The drawing under review shows one solid part. Ordinate dimensions are in mm from its lowest x, y, z. A direction names the side the tool comes from. Coordinates: 2 decimals unless noted, no trailing zeros. Write each loop counter-clockwise with the first axis right and the second up, starting at its lowest first coordinate (ties: lowest second). Pieces come first, ordered by that corner, then holes.
Q1. Insertion check: pin 1 (5 mm diameter, centred on x = 5.64, y = 5.64, fed in from -Z); pin 2 (2 mm diameter, centred on x = 2.5, z = 28.5, fed in from +Y); pin 3 (1.5 mm diameter, centred on y = 7.5, z = 12.5, fed in from -X). Each pin has a flat end and moves straight along its axis. Give the tip position at first contact, or say it passes through.
Q2. Take a section at B-B (y = 3.5). Give the boundary of the cut face in (x, z) (1 decimal), and give its area (3 significant figures).
Q3. Mouldability with a two-part tool opening along X and no side actions: class the marked faces 3, 4 and 5 as pulls with the +X half, pulls with the -X half, needs draft (parallel to the pull), parting line crosses it, or undercut.
Q4. Machinability: for the marked faces 1 and 2, which of the approach directions +Z, -Z, +X, -X, +Y, -Y give a long, thin tool a straight path to every point of the face, cutting with its end or side? Answer none if there is none.
Q5. Take a section at A-A (x = 7.25). Give the boundary of the cut face in (y, z) (1 decimal).
Q6. Take a section at D-D (z = 35). Give the boundary of the cut face in (x, y).
Q7. Take a section at C-C (z = 4.5). Give the boundary of the cut face in (x, y).
Q8. For probe 1 along Z at (x, y) = (0.75, 6.25); probe 2 along Z at (x, y) = (4.75, 7.5); probe 3 along Y at (x, z) = (6.75, 2), list the stretches that pass through material, from the lowest coordinate up.
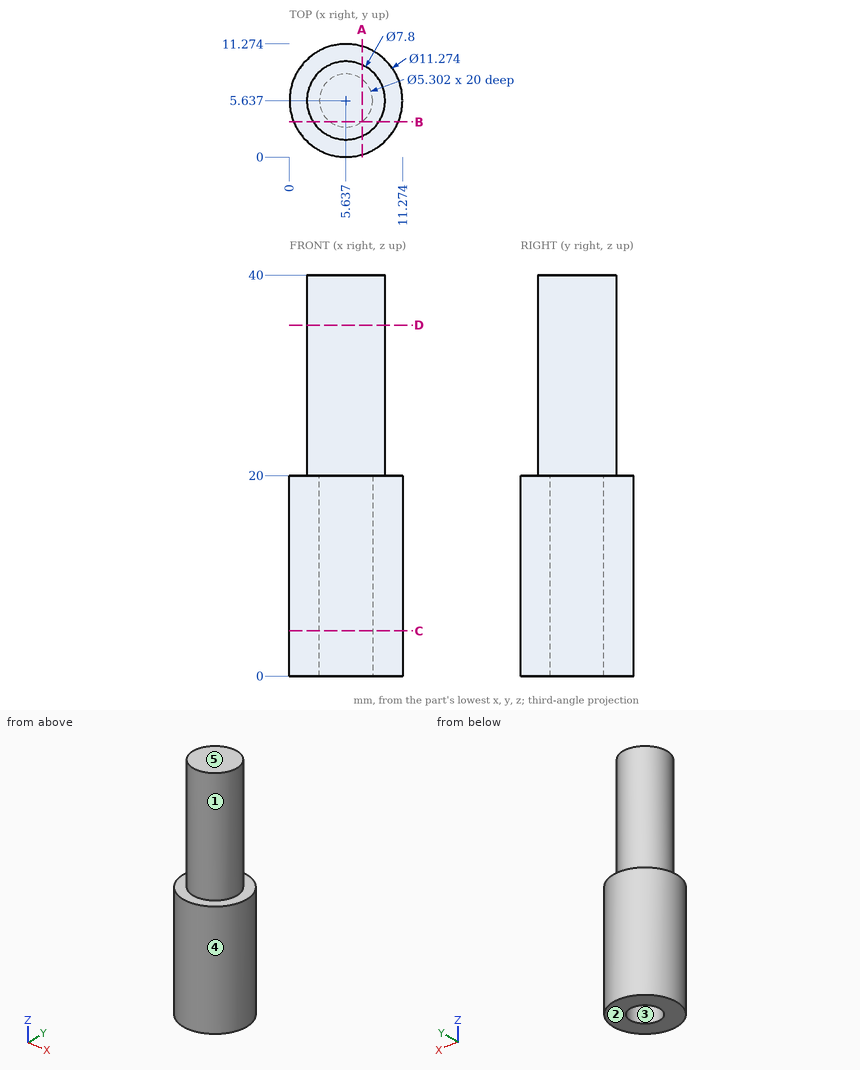
Response:
1. pin 1: stops at z = 20
1. pin 2: stops at y = 8.9
1. pin 3: stops at x = 0.11
2. outline: (0.4, 0) - (4.1, 0) - (4.1, 20) - (7.2, 20) - (7.2, 0) - (10.9, 0) - (10.9, 20) - (8.9, 20) - (8.9, 40) - (2.4, 40) - (2.4, 20) - (0.4, 20) - close
2. area: 276 mm2
3. face 3: undercut
3. face 4: parting line crosses it
3. face 5: needs draft
4. face 1: +Z
4. face 2: -Z, +X, -X, +Y, -Y
5. outline: (0.2, 0) - (3.5, 0) - (3.5, 20) - (7.7, 20) - (7.7, 0) - (11, 0) - (11, 20) - (9.2, 20) - (9.2, 40) - (2.1, 40) - (2.1, 20) - (0.2, 20) - close
6. outline: circle Ø7.8 at (5.64, 5.64)
7. outline: circle Ø11.27 at (5.64, 5.64); hole circle Ø5.3 at (5.64, 5.64)
8. probe 1: z = 0 to 20
8. probe 2: z = 20 to 40
8. probe 3: y = 0.11 to 3.23, 8.04 to 11.16
